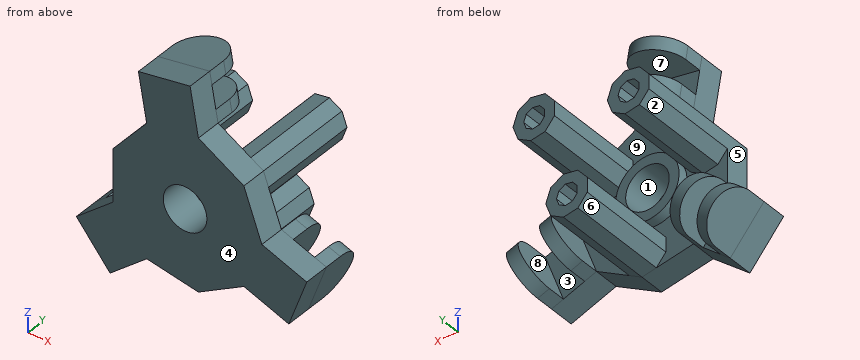
```python
from build123d import *

# Parameters (mm, degrees)
SKETCH1_R            = 5.5
BOSS_EXTRUDE1_DEPTH  = 6.35
BOSS_EXTRUDE2_DEPTH  = 3.18
BOSS_EXTRUDE4_DEPTH  = 3.175
BOSS_EXTRUDE5_DEPTH  = 3.175
BOSS_EXTRUDE6_DEPTH  = 3.175
BOSS_EXTRUDE7_DEPTH  = 3.175
BOSS_EXTRUDE8_DEPTH  = 3.175
BOSS_EXTRUDE9_DEPTH  = 25.4
SKETCH15_R           = 8
SKETCH15_R_2         = 5.5
BOSS_EXTRUDE10_DEPTH = 2.54


with BuildPart() as part:
    # Sketch1 → Boss-Extrude1 (new body)
    with BuildSketch(Plane(origin=(0, 0, 0), x_dir=(1, 0, 0), z_dir=(0, 1, 0))):
        Polygon((1.265828837, -30.968710893), (-11.781412955, -28.668130141), (-9.68401773, -16.773210729), (3.363224062, -19.073791481), align=None)
        Polygon((-9.68401773, -16.773210729), (3.363224062, -19.073791481), (14.836775938, -12.449533217), (19.368035459, 0), (14.836775938, 12.449533217), (3.363224062, 19.073791481), (-9.68401773, 16.773210729), (-18.2, 6.624258264), (-18.2, -6.624258264), align=None)
        Circle(SKETCH1_R, mode=Mode.SUBTRACT)
        Polygon((26.186775938, 16.580595376), (30.718035459, 4.131062159), (19.368035459, 0), (14.836775938, 12.449533217), align=None)
        Polygon((-27.452604774, 14.388115517), (-18.936622504, 24.537067982), (-9.68401773, 16.773210729), (-18.2, 6.624258264), align=None)
    extrude(amount=BOSS_EXTRUDE1_DEPTH)

    # Sketch4 → Boss-Extrude2 (add)
    with BuildSketch(Plane(origin=(-5.257792059, 0, 29.818420517), x_dir=(-0.984807753, 0, -0.173648178), z_dir=(0.173648178, 0, -0.984807753))):
        with BuildLine():
            Line((-6.624258264, 6.35), (-6.624258264, 10.84999989))
            ThreePointArc((-6.624258264, 10.84999989), (0, 17.474258154), (6.624258264, 10.84999989))
            Line((6.624258264, 10.84999989), (6.624258264, 6.35))
            Line((6.624258264, 6.35), (-6.624258264, 6.35))
        make_face()
    extrude(amount=BOSS_EXTRUDE2_DEPTH)

    # Sketch6 → Boss-Extrude4 (add)
    with BuildSketch(Plane(origin=(-3.160396834, 0, 17.923501105), x_dir=(-0.984807753, 0, -0.173648178), z_dir=(0.173648178, 0, -0.984807753))):
        with BuildLine():
            Line((-6.624258264, 6.35), (-6.624258264, 10.85))
            ThreePointArc((-6.624258264, 10.85), (0, 17.474258264), (6.624258264, 10.85))
            Line((6.624258264, 10.85), (6.624258264, 6.35))
            Line((6.624258264, 6.35), (-6.624258264, 6.35))
        make_face()
    extrude(amount=-BOSS_EXTRUDE4_DEPTH)

    # Sketch8 → Boss-Extrude5 (add)
    with BuildSketch(Plane(origin=(28.452405698, 0, -10.355828767), x_dir=(0.342020143, 0, 0.939692621), z_dir=(-0.939692621, 0, 0.342020143))):
        with BuildLine():
            Line((-6.624258264, 10.85), (-6.624258264, 6.35))
            Line((-6.624258264, 6.35), (6.624258264, 6.35))
            Line((6.624258264, 6.35), (6.624258264, 10.85))
            ThreePointArc((6.624258264, 10.85), (0, 17.474258264), (-6.624258264, 10.85))
        make_face()
    extrude(amount=BOSS_EXTRUDE5_DEPTH)

    # Sketch9 → Boss-Extrude6 (add)
    with BuildSketch(Plane(origin=(17.102405698, 0, -6.224766609), x_dir=(0.342020143, 0, 0.939692621), z_dir=(-0.939692621, 0, 0.342020143))):
        with BuildLine():
            Line((-6.624258264, 6.35), (-6.624258264, 10.85))
            ThreePointArc((-6.624258264, 10.85), (0, 17.474258264), (6.624258264, 10.85))
            Line((6.624258264, 10.85), (6.624258264, 6.35))
            Line((6.624258264, 6.35), (-6.624258264, 6.35))
        make_face()
    extrude(amount=-BOSS_EXTRUDE6_DEPTH)

    # Sketch10 → Boss-Extrude7 (add)
    with BuildSketch(Plane(origin=(-23.194613639, 0, -19.46259175), x_dir=(0.64278761, 0, -0.766044443), z_dir=(0.766044443, 0, 0.64278761))):
        with BuildLine():
            Line((-6.624258264, 10.85), (-6.624258264, 6.35))
            Line((-6.624258264, 6.35), (6.624258264, 6.35))
            Line((6.624258264, 6.35), (6.624258264, 10.85))
            ThreePointArc((6.624258264, 10.85), (0, 17.474258264), (-6.624258264, 10.85))
        make_face()
    extrude(amount=BOSS_EXTRUDE7_DEPTH)

    # Sketch11 → Boss-Extrude8 (add)
    with BuildSketch(Plane(origin=(-13.942008865, 0, -11.698734496), x_dir=(0.64278761, 0, -0.766044443), z_dir=(0.766044443, 0, 0.64278761))):
        with BuildLine():
            Line((-6.624258264, 10.85), (-6.624258264, 6.35))
            Line((-6.624258264, 6.35), (6.624258264, 6.35))
            Line((6.624258264, 6.35), (6.624258264, 10.85))
            ThreePointArc((6.624258264, 10.85), (0, 17.474258264), (-6.624258264, 10.85))
        make_face()
    extrude(amount=-BOSS_EXTRUDE8_DEPTH)

    # Sketch12 → Boss-Extrude9 (add)
    with BuildSketch(Plane(origin=(0, 6.35, 0), x_dir=(1, 0, 0), z_dir=(0, 1, 0))):
        Polygon((14.836775938, -12.449533217), (16.101545079, -8.974608561), (14.836775938, -5.499683905), (11.634268052, -3.650715115), (7.992510452, -4.292855237), (5.615521995, -7.125639771), (5.615521995, -10.823577351), (7.992510452, -13.656361885), (11.634268052, -14.298502007), align=None)
        Polygon((12.766148966, -10.712070889), (13.398533537, -8.974608561), (12.766148966, -7.237146233), (11.164895023, -6.312661838), (9.344016223, -6.633731899), (8.155521995, -8.050124166), (8.155521995, -9.899092956), (9.344016223, -11.315485223), (11.164895023, -11.636555284), align=None, mode=Mode.SUBTRACT)
        Polygon((6.565731948, 10.274973378), (7.83050109, 13.749898034), (6.565731948, 17.224822691), (3.363224062, 19.073791481), (-0.278533537, 18.431651359), (-2.655521995, 15.598866825), (-2.655521995, 11.900929244), (-0.278533537, 9.06814471), (3.363224062, 8.426004588), align=None)
        Polygon((-0.115521995, 12.825413639), (1.072972234, 11.409021372), (2.893851034, 11.087951311), (4.495104977, 12.012435706), (5.127489548, 13.749898034), (4.495104977, 15.487360363), (2.893851034, 16.411844758), (1.072972234, 16.090774697), (-0.115521995, 14.674382429), align=None, mode=Mode.SUBTRACT)
        Polygon((-18.2, -6.624258264), (-15.823011542, -9.457042798), (-12.181253943, -10.09918292), (-8.978746057, -8.25021413), (-7.713976916, -4.775289474), (-8.978746057, -1.300364817), (-12.181253943, 0.548603973), (-15.823011542, -0.093536149), (-18.2, -2.926320684), align=None)
        Polygon((-11.049373028, -6.512751802), (-10.416988458, -4.775289474), (-11.049373028, -3.037827145), (-12.650626972, -2.11334275), (-14.471505771, -2.434412811), (-15.66, -3.850805079), (-15.66, -5.699773869), (-14.471505771, -7.116166136), (-12.650626972, -7.437236197), align=None, mode=Mode.SUBTRACT)
    extrude(amount=BOSS_EXTRUDE9_DEPTH)

    # Sketch15 → Boss-Extrude10 (add)
    with BuildSketch(Plane(origin=(0, 6.35, 0), x_dir=(1, 0, 0), z_dir=(0, 1, 0))):
        Circle(SKETCH15_R)
        Circle(SKETCH15_R_2, mode=Mode.SUBTRACT)
    extrude(amount=BOSS_EXTRUDE10_DEPTH)


solid = part.part
```
Verification items for the finished model (mm, model axes). Face numbers are marked on the shaded views. A direction names the side the tool comes from. Give positions to 0.01 mm unless a question says otherwise; leave off trailing zeros. Order: outer loops, then holes, each group sorted by start corner. A loop starts at its lowest first (then second) coordinate and runs counter-clockwise, first axis right, second up. Notation, with made-up numbers: M 41,51.25 L 78,51.25 A25 cw 78,81.25 Z; hole C 32,84 d4. An arc over 180 degrees is marked long. Answer in a Markdown table with one row per item. Add a question column.
Item 1: Gauge pin test, flat ends, axial feed: pin 1 (4 mm diameter, centred on x = -1.5, z = 22, fed in from +Y); pin 2 (8 mm diameter, centred on y = 13.5, z = 12, fed in from -X); pin 3 (0.9 mm diameter, centred on y = 13, z = 4.5, fed in from +X). Record the tip position at first contact, or that the pin passes through.
Item 2: Section check B-B, the plane y = 28. State how many separate pieces and enclosed holes the cut face has, and give its area (3 significant figures).
Item 3: Mould release check, pull along X, two halves, no side actions. Record for the marked faces 1, 2, 3 and 4: released by +X, released by -X, zero draft, split by the parting line, or undercut.
Item 4: Tool access check on the marked faces 5, 6, 7, 8 and 9. Record the directions out of +Z, -Z, +X, -X, +Y, -Y that give a thin tool (end or side, any length) a straight path to the whole face; none if there is none.
Item 5: Scan lines: probe 1 along Z at (x, y) = (-9, 28); probe 2 along X at (y, z) = (13, -11); probe 3 along Y at (x, z) = (11, -2). Record each from-to range of solid material in increasing order. Write a range as from..to.
Item 6: Section check A-A, the plane y = 3.5. Enter the section's corners in (x, z), and give its area (3 significant figures).
Filled sheet:
| question | item | result |
|---|---|---|
| 1 | pin 1 | stops at y = 17.46 |
| 1 | pin 2 | stops at x = -17.05 |
| 1 | pin 3 | stops at x = 13.88 |
| 2 | separate pieces | 3 |
| 2 | enclosed holes | 3 |
| 2 | area | 190 mm^2 |
| 3 | face 1 | undercut |
| 3 | face 2 | released by -X |
| 3 | face 3 | undercut |
| 3 | face 4 | zero draft |
| 4 | face 5 | +Z, -X, +Y, -Y |
| 4 | face 6 | -Z, +Y |
| 4 | face 7 | +X, +Y |
| 4 | face 8 | +Z, +Y |
| 4 | face 9 | +Y |
| 5 | probe 1 | z = 1.29..8.26 |
| 5 | probe 2 | x = -18.67..-14.53, -1.9..6.83, 15.36..18.74, 24.84..28.22 |
| 5 | probe 3 | y = 0..6.35 |
| 6 | outline | M -27.45,-14.39 L -18.94,-24.54 L -9.68,-16.77 L 3.36,-19.07 L 14.84,-12.45 L 26.19,-16.58 L 30.72,-4.13 L 19.37,0 L 14.84,12.45 L 3.36,19.07 L 1.27,30.97 L -11.78,28.67 L -9.68,16.77 L -18.2,6.62 L -18.2,-6.62 Z; hole C 0,0 d11 |
| 6 | area | 1,470 mm^2 |
